Design review of the part shown in the three views and the two pictorial views. Dimensions are in mm from the part's minimum x, y and z. A direction names the side the tool comes from. Round coordinates to 2 decimals unless told otherwise and drop trailing zeros. Order: outer loops, then holes, each group sorted by start corner. A loop starts at its lowest first (then second) coordinate and runs counter-clockwise, first axis right, second up. Notation, with made-up numbers: M 45,-24.5 L 51,-24.5 A20 cw 51,-6.5 Z; hole C 62,9 d6. An arc over 180 degrees is marked long. Write item = value, one per line. Start each with the question number.
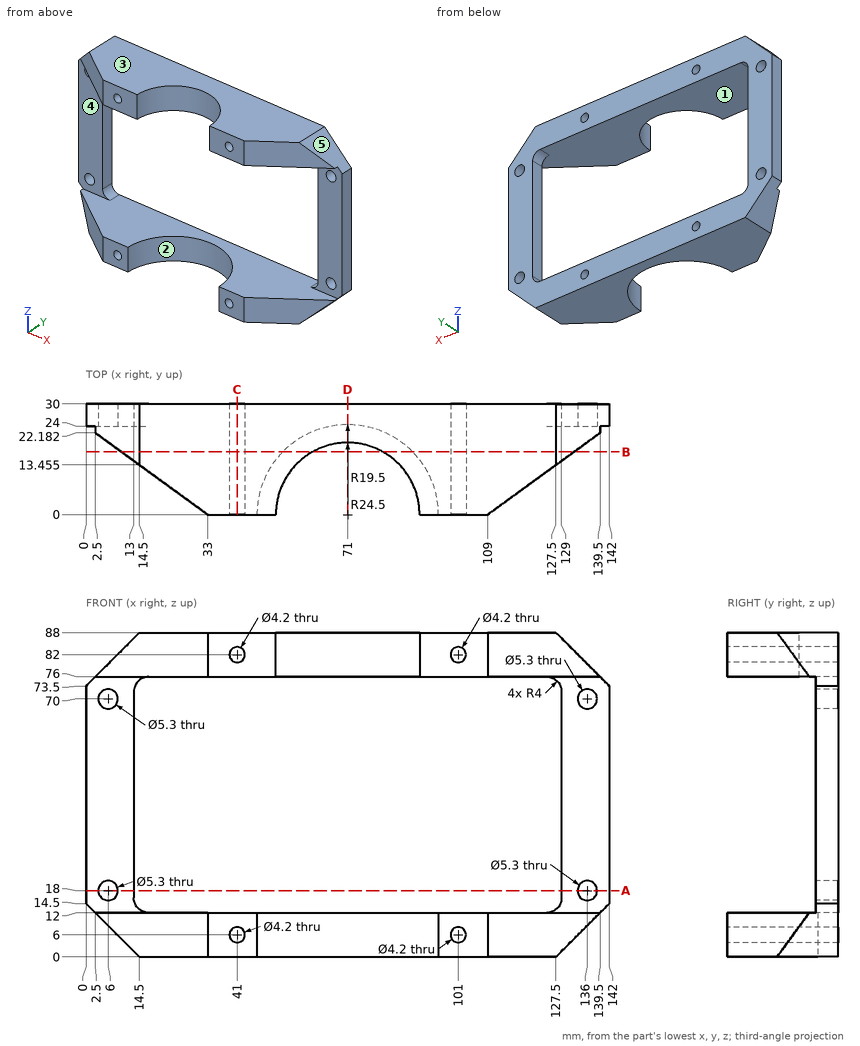
(1) We need section D-D, the plane x = 71. Write out the cut boundary in (y, z).
(2) Draft analysis for pull direction Z (two halves, no side actions). For the marked faces 1, 2 and 3, state which applies: released by +Z, released by -Z, zero draft, split by the parting line, or undercut.
(3) We need section B-B, the plane y = 17. Write out the cut boundary in (x, z) (1 decimal), then the cut area to 3 significant figures.
(4) We need section C-C, the plane x = 41. Write out the cut boundary in (y, z), then the cut area to 3 significant figures.
(5) We need section A-A, the plane z = 18. Write out the cut boundary in (x, y).
(6) Insertion check: pin 1 (4 mm diameter, centred on x = 53, z = 9, fed in from -Y); pin 2 (5 mm diameter, centred on x = 41, z = 82, fed in from -Y); pin 3 (15 mm diameter, centred on x = 79.5, y = 14.5, fed in from -Z); pin 4 (13.5 mm diameter, centred on x = 129.5, z = 35.5, fed in from -Y). Each pin has a flat end and moves straight along its axis. Give the tip position at first contact, or say it passes through.
(7) For the marked faces 4 and 5, list the 3-axis set-ups (+Z, -Z, +X, -X, +Y, -Y) from which the entire face can be reached by the end or side of a thin tool; tool diameter is ignored.
(8) For line 1 along Z through (x, y) = (41, 22.5); line 2 along Z through (x, y) = (111, 26.5); line 3 along Z through (x, y) = (136, 28.5), list the stretches that pass through material, from the lowest coordinate up.
Values:
q1.outline = M 19.5,76 L 30,76 L 30,88 L 19.5,88 Z; M 24.5,0 L 30,0 L 30,12 L 24.5,12 Z
q2.face_1 = undercut
q2.face_2 = zero draft
q2.face_3 = released by +Z
q3.outline = M 9.6,4.9 L 14.5,0 L 53.4,0 L 53.4,12 L 9.6,12 Z; M 9.6,76 L 61.4,76 L 61.4,88 L 14.5,88 L 9.6,83.1 Z; M 80.6,76 L 132.4,76 L 132.4,83.1 L 127.5,88 L 80.6,88 Z; M 88.6,0 L 127.5,0 L 132.4,4.9 L 132.4,12 L 88.6,12 Z; hole C 41,6 d4.2; hole C 41,82 d4.2; hole C 101,6 d4.2; hole C 101,82 d4.2
q3.area = 2,190 mm²
q4.outline = M 0,0 L 30,0 L 30,3.9 L 0,3.9 Z; M 0,8.1 L 30,8.1 L 30,12 L 0,12 Z; M 0,76 L 30,76 L 30,79.9 L 0,79.9 Z; M 0,84.1 L 30,84.1 L 30,88 L 0,88 Z
q4.area = 468 mm²
q5.outline = M 0,24 L 3.35,24 L 3.35,30 L 0,30 Z; M 8.65,24 L 13,24 L 13,30 L 8.65,30 Z; M 129,24 L 133.35,24 L 133.35,30 L 129,30 Z; M 138.65,24 L 142,24 L 142,30 L 138.65,30 Z
q6.pin_1 = 14.15
q6.pin_2 = 0
q6.pin_3 = 76
q6.pin_4 = 24
q7.face_4 = +X, -X, -Y
q7.face_5 = +Z, +X, +Y, -Y
q8.line_1 = 0 to 3.9, 8.1 to 12, 76 to 79.9, 84.1 to 88
q8.line_2 = 0 to 12, 76 to 88
q8.line_3 = 8.5 to 15.35, 20.65 to 67.35, 72.65 to 79.5
